```python
from build123d import *

# Parameters (mm, degrees)
BOSS_EXTRUDE1_DEPTH = 8
SKETCH2_R           = 1.35
CUT_EXTRUDE1_DEPTH  = 10
CUT_EXTRUDE2_REACH  = 7
SKETCH4_R           = 2.6


with BuildPart() as part:
    # Sketch1 → Boss-Extrude1 (new body)
    with BuildSketch(Plane(origin=(0, 0, 0), x_dir=(1, 0, 0), z_dir=(0, 1, 0))):
        Polygon((0, 0), (0, 26), (7, 26), (7, 5), (25, 5), (25, 0), align=None)
    extrude(amount=BOSS_EXTRUDE1_DEPTH)

    # Sketch2 → Cut-Extrude1 (cut)
    with BuildSketch(Plane.ZY):
        with Locations((-23, 2.75)):
            Circle(SKETCH2_R)
        with Locations((-3.5, 2.75)):
            Circle(SKETCH2_R)
    extrude(amount=-CUT_EXTRUDE1_DEPTH, mode=Mode.SUBTRACT)

    # Sketch4 → Cut-Extrude2 (cut, up to next)
    with BuildSketch(Plane(origin=(0, 0, -5), x_dir=(-1, 0, 0), z_dir=(0, 0, -1)), mode=Mode.PRIVATE) as cut_extrude2_sk1:
        with Locations((-17, 4)):
            Circle(SKETCH4_R)
    cut_extrude2_tool1 = extrude(cut_extrude2_sk1.sketch, amount=-CUT_EXTRUDE2_REACH, mode=Mode.PRIVATE) & part.part
    add(cut_extrude2_tool1.solids().sort_by_distance((17, 4, -5))[0], mode=Mode.SUBTRACT)


solid = part.part
```
For this review, take the finished solid that the model builds, in its own axes (mm). A direction names the side the tool comes from. Round coordinates to 2 decimals unless told otherwise and drop trailing zeros. Loops run counter-clockwise (first coordinate to the right, second up) from the corner with the lowest first, then second, coordinate; pieces in that order, holes last.
(1) Mouldability with a two-part tool opening along X and no side actions: class faces 4 (the flat face through (10, 3, -4)), 5 (the flat face through (25, 4, -3)), 6 (the flat face through (14, 4, -5)), 7 (the cylindrical face through (14.52, 4.78, -2.54)) as released by +X, released by -X, zero draft, split by the parting line, or undercut.
Returned:
face 4: released by -X
face 5: released by +X
face 6: zero draft
face 7: undercut
(2) We need section A-A (x = 17). Give the boundary of the cut face in (y, z), plus the area to 3 significant figures.
Returned:
outline: (0, -5) - (1.4, -5) - (1.4, 0) - (0, 0) - close; (6.6, -5) - (8, -5) - (8, 0) - (6.6, 0) - close
area: 14.0 mm2
(3) Tool access review of faces 1 (the cylindrical face through (4.93, 1.55, -2.88)), 2 (the flat face through (4, 8, -7)), 3 (the flat face through (7, 4, -16)): name each direction out of +Z, -Z, +X, -X, +Y, -Y from which nothing blocks a thin tool from reaching the whole face with its end or side.
Returned:
face 1: -X
face 2: +Z, -Z, +X, -X, +Y
face 3: -Z, +X, +Y, -Y
(4) We need section C-C (z = -23). Give the boundary of the cut face in (x, y).
Returned:
outline: (0, 0) - (7, 0) - (7, 1.4) - (0, 1.4) - close; (0, 4.1) - (7, 4.1) - (7, 8) - (0, 8) - close
(5) We need section D-D (y = 1.75). Give the boundary of the cut face in (x, z), plus the area to 3 significant figures.
Returned:
outline: (0, -26) - (7, -26) - (7, -23.91) - (0, -23.91) - close; (0, -22.09) - (7, -22.09) - (7, -5) - (15.7, -5) - (15.7, 0) - (0, 0) - (0, -2.59) - (10, -2.59) - (10, -4.41) - (0, -4.41) - close; (18.3, -5) - (25, -5) - (25, 0) - (18.3, 0) - close
area: 228 mm2
(6) Wall thickness on line 1 along Y through (x, z) = (6.75, -3.5); line 2 along X through (y, z) = (0.75, -16.25); line 3 along Y through (x, z) = (8, -2.5): over which ranges is each line inside the solid? List them lowest first.
Returned:
line 1: y = 0 to 1.4, 4.1 to 8
line 2: x = 0 to 7
line 3: y = 0 to 1.84, 3.66 to 8
(7) Clearance check with flat-ended pins moving along their axes: P1, Ø2.5, axis at x = 14.5, y = 4.5, coming from the -Z side; P2, Ø3.5, axis at y = 2.75, z = -23, coming from the +X side; P3, Ø0.8, axis at y = 3, z = -4, coming from the -X side; P4, Ø1.5, axis at x = 13.5, z = -6.5, coming from the -Y side. State where each tip first meets the part, or that it passes through.
Returned:
P1: stops at z = -5
P2: stops at x = 7
P3: stops at x = 10
P4: passes through
(8) We need section B-B (y = 5). Give the boundary of the cut face in (x, z), plus the area to 3 significant figures.
Returned:
outline: (0, -26) - (7, -26) - (7, -5) - (14.6, -5) - (14.6, 0) - (0, 0) - close; (19.4, -5) - (25, -5) - (25, 0) - (19.4, 0) - close
area: 248 mm2
